```python
from build123d import *

# Parameters (mm, degrees)
SKETCH1_R           = 4
BOSS_EXTRUDE1_DEPTH = 20


with BuildPart() as part:
    # Sketch1 → Boss-Extrude1 (new body)
    with BuildSketch(Plane(origin=(0, 0, 0), x_dir=(1, 0, 0), z_dir=(0, 1, 0))):
        with Locations(Location((0, 0, 0), (0, 0, 270))):
            Circle(SKETCH1_R)
        with BuildLine():
            ThreePointArc((-2.5, 2.5), (-1.464466094, 0), (-2.5, -2.5))
            ThreePointArc((-2.5, -2.5), (0, -1.464466094), (2.5, -2.5))
            ThreePointArc((2.5, -2.5), (1.464466094, 0), (2.5, 2.5))
            ThreePointArc((2.5, 2.5), (0, 1.464466094), (-2.5, 2.5))
        make_face(mode=Mode.SUBTRACT)
    extrude(amount=BOSS_EXTRUDE1_DEPTH)


solid = part.part
```
Build history of the part. All positions in model axes, mm. Round coordinates to 2 decimals unless told otherwise and drop trailing zeros. Write each loop counter-clockwise with the first axis right and the second up, starting at its lowest first coordinate (ties: lowest second). Pieces come first, ordered by that corner, then holes.
1) Band-saw the part on D-D, the plane z = -2. List the corners of the cut face in (x, y).
2) Band-saw the part on C-C, the plane y = 1.5. List the corners of the cut face in (x, z), and give its area (3 significant figures).
3) Band-saw the part on B-B, the plane z = 0. List the corners of the cut face in (x, y).
4) Drill centre lines: probe 1 along X at (y, z) = (9.5, 0); probe 2 along Z at (x, y) = (-1.75, 16.25); probe 3 along Z at (x, y) = (1, 7.5). Where is each one in solid material? Low to high.
5) Mould opens along X. For faces 1 (the cylindrical face through (-0.039, 9.86, 1.465)), 2 (the flat face through (0, 0, 2)), 3 (the cylindrical face through (-3.905, 9.86, -0.867)) say: +X half, -X half, draft (parallel to the pull), parting line (faces both ways), or undercut.
6) Pin check, flat tips, straight feed: pin 1 (1.5 mm diameter, centred on x = -3, z = 0.5, fed in from -Y); pin 2 (1 mm diameter, centred on y = 15, z = 1, fed in from -X); pin 3 (1.5 mm diameter, centred on y = 9, z = 2, fed in from -X). Stop position of each tip, or through.
7) Band-saw the part on A-A, the plane x = 0. List the corners of the cut face in (y, z).
Ans:
1. outline: (-3.46, 0) - (-2.08, 0) - (-2.08, 20) - (-3.46, 20) - close; (-1.87, 0) - (1.87, 0) - (1.87, 20) - (-1.87, 20) - close; (2.08, 0) - (3.46, 0) - (3.46, 20) - (2.08, 20) - close
2. outline: circle Ø8 at (0, 0); hole (-2.5, -2.5) arc R3.54 cw to (2.5, -2.5) arc R3.54 cw to (2.5, 2.5) arc R3.54 cw to (-2.5, 2.5) arc R3.54 cw to start
2. area: 39.5 mm2
3. outline: (-4, 0) - (-1.46, 0) - (-1.46, 20) - (-4, 20) - close; (1.46, 0) - (4, 0) - (4, 20) - (1.46, 20) - close
4. probe 1: x = -4 to -1.46, 1.46 to 4
4. probe 2: z = -3.6 to -1.93, -1.39 to 1.39, 1.93 to 3.6
4. probe 3: z = -3.87 to -1.61, 1.61 to 3.87
5. face 1: undercut
5. face 2: draft
5. face 3: parting line
6. pin 1: stops at y = 0
6. pin 2: stops at x = -3.97
6. pin 3: stops at x = -3.8
7. outline: (0, -4) - (20, -4) - (20, -1.46) - (0, -1.46) - close; (0, 1.46) - (20, 1.46) - (20, 4) - (0, 4) - close
